from build123d import *

# Parameters (mm, degrees)
SKETCH1_W            = 3
SKETCH1_H            = 14
BOSS_EXTRUDE1_DEPTH  = 14
SKETCH2_R            = 0.65
CUT_EXTRUDE1_DEPTH   = 21.024984395
M2_CLEARANCE_HOLE1_D = 2.4


with BuildPart() as part:
    # Sketch1 → Boss-Extrude1 (new body)
    with BuildSketch(Plane(origin=(0, 0, 0), x_dir=(1, 0, 0), z_dir=(0, 1, 0))):
        with Locations((1.5, -7)):
            Rectangle(SKETCH1_W, SKETCH1_H)
    extrude(amount=BOSS_EXTRUDE1_DEPTH)

    # Sketch2 → Cut-Extrude1 (cut, through all)
    with BuildSketch(Plane(origin=(0, 0, 0), x_dir=(1, 0, 0), z_dir=(0, 1, 0))):
        Circle(SKETCH2_R)
        with Locations((0, -2)):
            Circle(SKETCH2_R)
        with Locations((0, -4)):
            Circle(SKETCH2_R)
        with Locations((0, -6)):
            Circle(SKETCH2_R)
        with Locations((0, -8)):
            Circle(SKETCH2_R)
        with Locations((0, -10)):
            Circle(SKETCH2_R)
        with Locations((0, -12)):
            Circle(SKETCH2_R)
        with Locations((0, -14)):
            Circle(SKETCH2_R)
    extrude(amount=CUT_EXTRUDE1_DEPTH, mode=Mode.SUBTRACT)

    # M2 Clearance Hole1 (through all)
    with Locations(Plane(origin=(3, 0, 0), x_dir=(0, 0, -1), z_dir=(1, 0, 0))):
        with Locations((-7, 12), (-7, 2)):
            Hole(M2_CLEARANCE_HOLE1_D / 2)


solid = part.part
Input: part model. Units: mm. Frame: model coordinates. Coordinates: 2 decimals unless noted, no trailing zeros. Order: outer loops, then holes, each group sorted by start corner. A loop starts at its lowest first (then second) coordinate and runs counter-clockwise, first axis right, second up. Notation, with made-up numbers: M 88,27.5 L 107,27.5 A15 cw 107,52.5 Z; hole C 9.5,36 d8. An arc over 180 degrees is marked long. One line per question, with ' | ' between items.
Item 1: Section C-C (y = 2.5). Output: boundary loops of the cut face in (x, z), then the cut area to 3 significant figures.
Geometry results:
outline: M 0,0.65 A0.65 cw 0.65,0 L 3,0 L 3,5.91 L 0.64,5.91 A0.65 cw 0,5.35 L 0,4.65 A0.65 cw 0,3.35 L 0,2.65 A0.65 cw 0,1.35 Z; M 0,8.65 A0.65 cw 0.64,8.09 L 3,8.09 L 3,14 L 0.65,14 A0.65 cw 0,13.35 L 0,12.65 A0.65 cw 0,11.35 L 0,10.65 A0.65 cw 0,9.35 Z | area: 31.6 mm^2
Item 2: Section B-B (x = 1.85). Output: boundary loops of the cut face in (y, z), then the cut area to 3 significant figures.
Geometry results:
outline: M 0,0 L 14,0 L 14,14 L 0,14 Z; hole C 2,7 d2.4; hole C 12,7 d2.4 | area: 187 mm^2
Item 3: Section D-D (y = 4.25). Output: boundary loops of the cut face in (x, z).
Geometry results:
outline: M 0,0.65 A0.65 cw 0.65,0 L 3,0 L 3,14 L 0.65,14 A0.65 cw 0,13.35 L 0,12.65 A0.65 cw 0,11.35 L 0,10.65 A0.65 cw 0,9.35 L 0,8.65 A0.65 cw 0,7.35 L 0,6.65 A0.65 cw 0,5.35 L 0,4.65 A0.65 cw 0,3.35 L 0,2.65 A0.65 cw 0,1.35 Z
Item 4: Section A-A (z = 7). Output: boundary loops of the cut face in (x, y), then the cut area to 3 significant figures.
Geometry results:
outline: M 0,0 L 3,0 L 3,0.8 L 0,0.8 Z; M 0,3.2 L 3,3.2 L 3,10.8 L 0,10.8 Z; M 0,13.2 L 3,13.2 L 3,14 L 0,14 Z | area: 27.6 mm^2
Item 5: Ray query, line 1 along Y through (x, z) = (1.9, 7); line 2 along Z through (x, y) = (1.7, 2); line 3 along X through (y, z) = (5.25, 12). Return the intervals inside material, ascending.
Geometry results:
line 1: y = 0 to 0.8, 3.2 to 10.8, 13.2 to 14 | line 2: z = 0 to 5.8, 8.2 to 14 | line 3: x = 0.65 to 3
Item 6: Draft query along Z for faces 1 (the flat face through (2, 7, 14)), 2 (the flat face through (2, 7, 0)), 3 (the cylindrical face through (0.65, 6.9, 8.01)). Return one class per face: released by +Z, released by -Z, zero draft, split by the parting line, or undercut.
Geometry results:
face 1: released by +Z | face 2: released by -Z | face 3: undercut
Item 7: Pin query (flat end, axial travel): pin 1 (1.4 mm diameter, centred on y = 12, z = 7, fed in from -X). Return the tip coordinate at first contact, or that it passes through.
Geometry results:
pin 1: passes through
